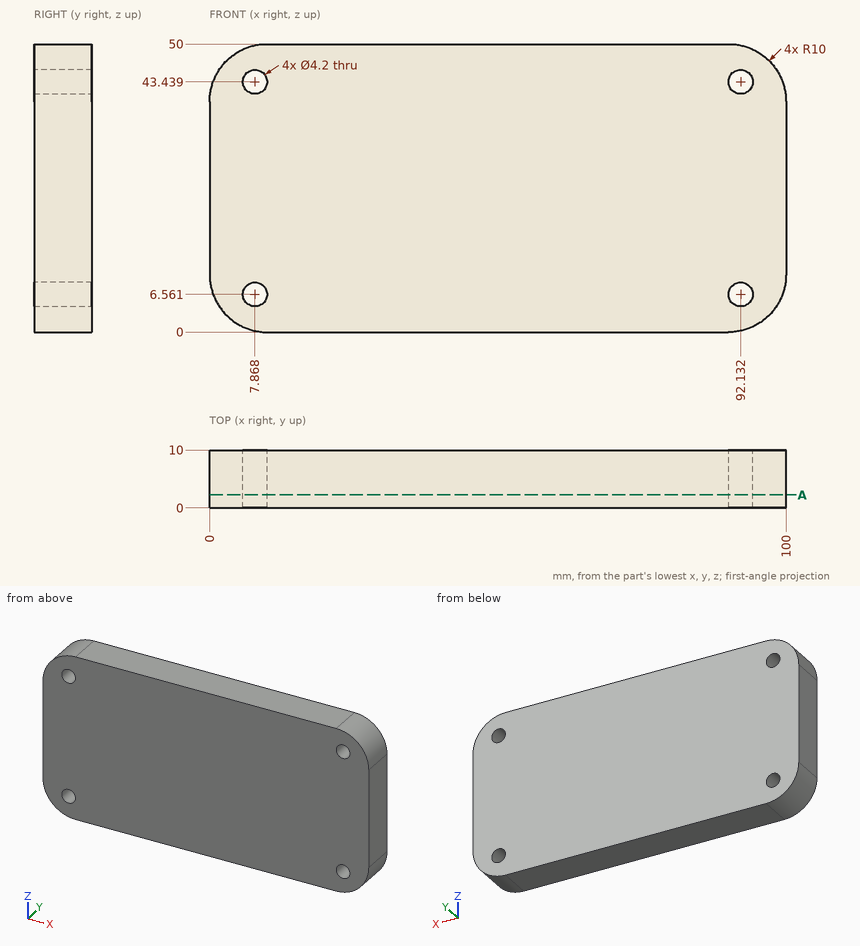
Study the drawing (mm; zero at the part's minimum x, y, z) and answer. Round coordinates to 2 decimals unless told otherwise and drop trailing zeros. Write each loop counter-clockwise with the first axis right and the second up, starting at its lowest first coordinate (ties: lowest second). Pieces come first, ordered by that corner, then holes. Notation, with made-up numbers: (80.25, 83) -> (114.25, 83) arc R34 cw to (114.25, 114) -> close; hole circle Ø6 at (-21.75, 26). An arc over 180 degrees is marked (long way). Answer as CSV lines item,"result". Start each with the question number.
(1) Find the intervals of material crossed by probe 1 along X at (y, z) = (2.25, 43) (1 decimal); probe 2 along Z at (x, y) = (8, 7.5) (1 decimal); probe 3 along X at (y, z) = (8.5, 46), in increasing order.
(2) The part is cut by section A-A, the plane y = 2.25. Give the vertices of the cut face in (x, z).
(3) This flat-tipped pin is pushed along its axis until it touches: pin 1 (2 mm diameter, centred on y = 6.5, z = 5.5, fed in from +X). Where does it stop, or does it pass through?
Output values:
1,probe 1,"x = 0.5 to 5.8, 9.9 to 90.1, 94.2 to 99.5"
1,probe 2,"z = 0.2 to 4.5, 8.7 to 41.3, 45.5 to 49.8"
1,probe 3,"x = 2 to 98"
2,outline,"(0, 10) arc R10 ccw to (10, 0) -> (90, 0) arc R10 ccw to (100, 10) -> (100, 40) arc R10 ccw to (90, 50) -> (10, 50) arc R10 ccw to (0, 40) -> close; hole circle Ø4.2 at (7.87, 6.56); hole circle Ø4.2 at (7.87, 43.44); hole circle Ø4.2 at (92.13, 6.56); hole circle Ø4.2 at (92.13, 43.44)"
3,pin 1,"stops at x = 99.37"
